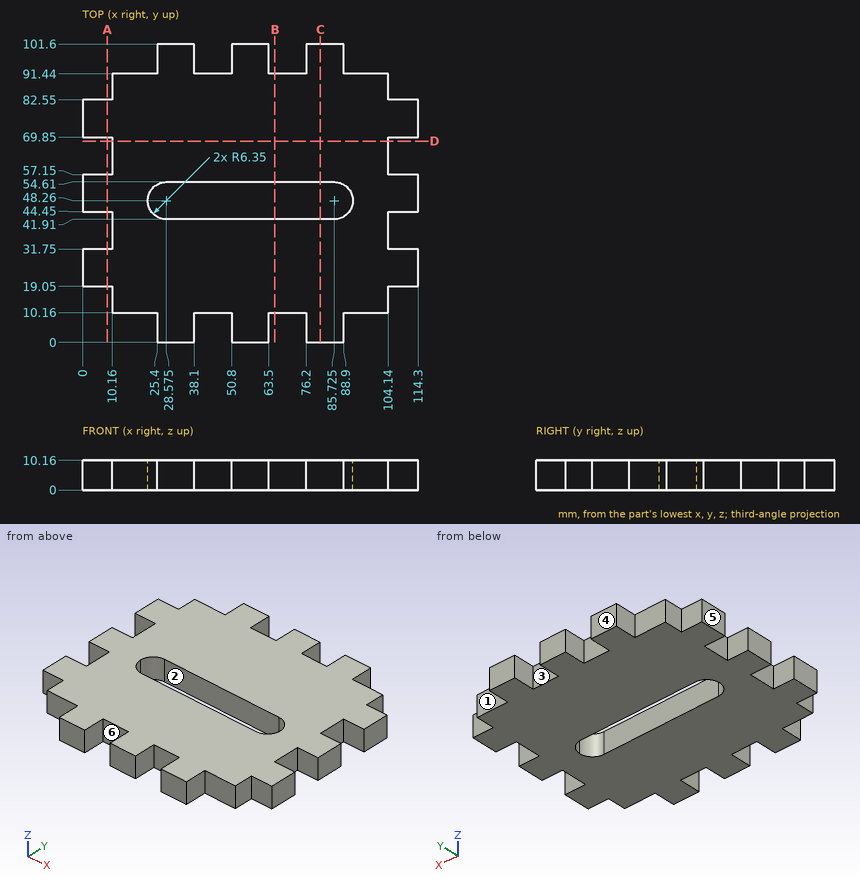
Study the drawing (mm; zero at the part's minimum x, y, z) and answer. A direction names the side the tool comes from. Coordinates: 2 decimals unless noted, no trailing zeros. Loops run counter-clockwise (first coordinate to the right, second up) from the corner with the lowest first, then second, coordinate; pieces in that order, holes last. Notation, with made-up numbers: M -25,56 L 18,56 A16 cw 18,73 Z; hole C 44.25,80.25 d4. An arc over 180 degrees is marked long. Answer in a Markdown table with one row per item.
1) Find section C-C (x = 81). Determine the outline of the cut face in (y, z).
Answers below:
| item | result |
|---|---|
| outline | M 0,0 L 41.91,0 L 41.91,10.16 L 0,10.16 Z; M 54.61,0 L 101.6,0 L 101.6,10.16 L 54.61,10.16 Z |
2) Given pin 1 (5 mm diameter, centred on x = 3.5, z = 4, fed in from -Y); pin 2 (3 mm diameter, centred on y = 2.5, z = 6.5, fed in from +X); pin 3 (5 mm diameter, centred on y = 86.5, z = 5, fed in from -X), each flat-ended and moving along its own axis, determine where each tip first touches the part or whether it passes through.
Answers below:
| item | result |
|---|---|
| pin 1 | y = 19.05 |
| pin 2 | x = 88.9 |
| pin 3 | x = 10.16 |
3) Find the intervals of material crossed by probe 1 along Y at (x, z) = (6.5, 6); probe 2 along Y at (x, z) = (84, 9); probe 3 along Y at (x, z) = (47.5, 7.5), in increasing order.
Answers below:
| item | result |
|---|---|
| probe 1 | 19.05 to 31.75, 44.45 to 57.15, 69.85 to 82.55 |
| probe 2 | 0 to 41.91, 54.61 to 101.6 |
| probe 3 | 10.16 to 41.91, 54.61 to 91.44 |
4) Find section A-A (x = 8.5). Determine the outline of the cut face in (y, z), then the cut area to 3 significant figures.
Answers below:
| item | result |
|---|---|
| outline | M 19.05,0 L 31.75,0 L 31.75,10.16 L 19.05,10.16 Z; M 44.45,0 L 57.15,0 L 57.15,10.16 L 44.45,10.16 Z; M 69.85,0 L 82.55,0 L 82.55,10.16 L 69.85,10.16 Z |
| area | 387 mm^2 |
5) Find section B-B (x = 65.5). Determine the outline of the cut face in (y, z), then the cut area to 3 significant figures.
Answers below:
| item | result |
|---|---|
| outline | M 10.16,0 L 41.91,0 L 41.91,10.16 L 10.16,10.16 Z; M 54.61,0 L 91.44,0 L 91.44,10.16 L 54.61,10.16 Z |
| area | 697 mm^2 |
6) Which of the six approach directions +Z, -Z, +X, -X, +Y, -Y give full straight-line access (tool end or side, diameter ignored) to the marked faces 1, 2 and 3?
Answers below:
| item | result |
|---|---|
| face 1 | +Z, -Z, +X, +Y |
| face 2 | +Z, -Z |
| face 3 | +Z, -Z, +Y |
7) Determine the mould class of the marked faces 4, 5 and 6 for opening direction X: released by +X, released by -X, zero draft, split by the parting line, or undercut.
Answers below:
| item | result |
|---|---|
| face 4 | zero draft |
| face 5 | released by -X |
| face 6 | undercut |
8) Find section D-D (y = 68.5). Determine the outline of the cut face in (x, z), then the cut area to 3 significant figures.
Answers below:
| item | result |
|---|---|
| outline | M 10.16,0 L 104.14,0 L 104.14,10.16 L 10.16,10.16 Z |
| area | 955 mm^2 |
